Geometry: see drawing. Coordinates: mm, zero at the bounding-box minimum. Coordinates: 2 decimals unless noted, no trailing zeros. Write each loop counter-clockwise with the first axis right and the second up, starting at its lowest first coordinate (ties: lowest second). Pieces come first, ordered by that corner, then holes. Notation, with made-up numbers: (37, 53.25) - (53, 53.25) arc R25 cw to (53, 66.25) - close; hole circle Ø4 at (11.25, 1.25). An arc over 180 degrees is marked (long way). One line per question, with ' | ' between items. Start each with the question number.
1) Section query B-B on y = 1.8. Return loops of the section in (x, z).
2) Line query: line 1 (Z direction, x = 9, y = 3.4); line 2 (X direction, y = 4.7, z = 3); line 3 (Z direction, x = 44.5, y = 3.35). Output: solid intervals per line, ascending.
3) Section query D-D on x = 36.5. Return loops of the section in (y, z), and give its area (3 significant figures).
4) Section query A-A on x = 10. Return loops of the section in (y, z), and give its area (3 significant figures).
5) First-contact query: P1, Ø1.5, axis at y = 2.5, z = 34.5, coming from the -X side; P2, Ø2.5, axis at y = 2.5, z = 22, coming from the +X side. Flat tips, straight axial feed; report the tip coordinate or a pass-through.
6) Section query C-C on z = 28.5. Return loops of the section in (x, y), and give its area (3 significant figures).
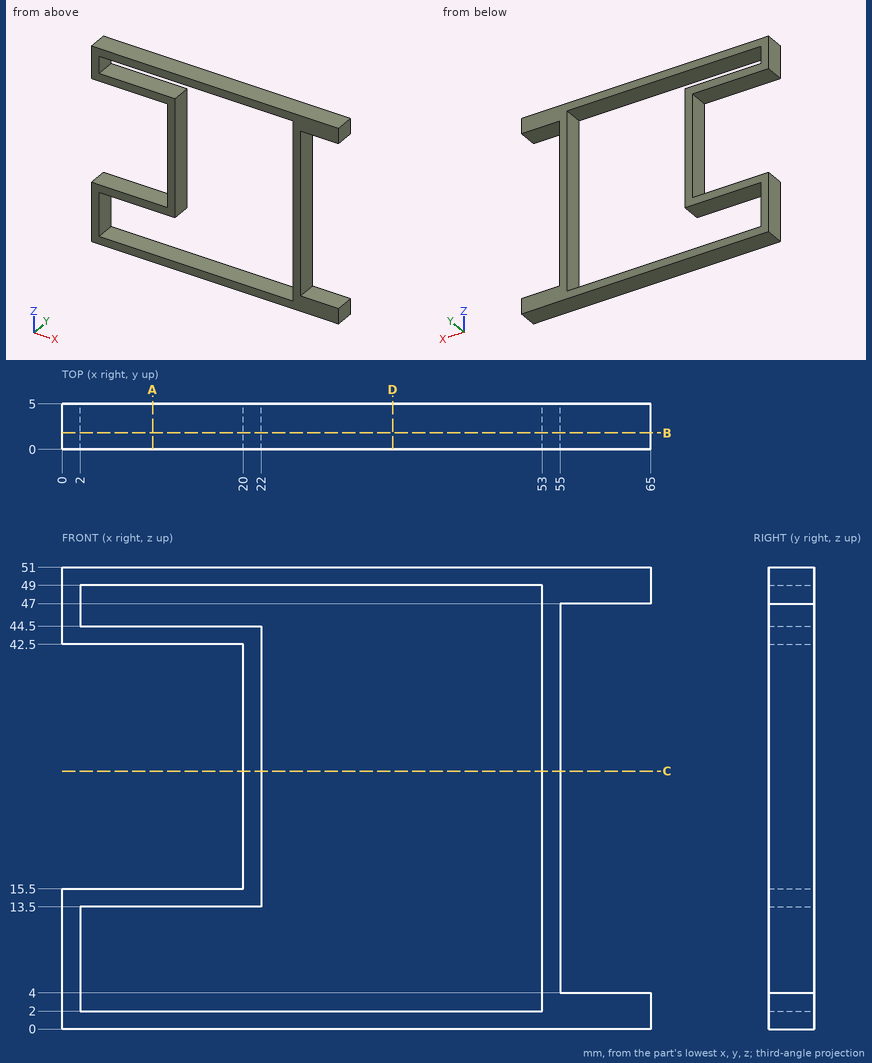
Answer key:
1) outline: (0, 0) - (65, 0) - (65, 4) - (55, 4) - (55, 47) - (65, 47) - (65, 51) - (0, 51) - (0, 42.5) - (20, 42.5) - (20, 15.5) - (0, 15.5) - close; hole (2, 2) - (53, 2) - (53, 49) - (2, 49) - (2, 44.5) - (22, 44.5) - (22, 13.5) - (2, 13.5) - close
2) line 1: 0 to 2, 13.5 to 15.5, 42.5 to 44.5, 49 to 51 | line 2: 0 to 2, 53 to 65 | line 3: 0 to 2, 49 to 51
3) outline: (0, 0) - (5, 0) - (5, 2) - (0, 2) - close; (0, 49) - (5, 49) - (5, 51) - (0, 51) - close | area: 20.0 mm²
4) outline: (0, 0) - (5, 0) - (5, 2) - (0, 2) - close; (0, 13.5) - (5, 13.5) - (5, 15.5) - (0, 15.5) - close; (0, 42.5) - (5, 42.5) - (5, 44.5) - (0, 44.5) - close; (0, 49) - (5, 49) - (5, 51) - (0, 51) - close | area: 40.0 mm²
5) P1: x = 20 | P2: x = 55
6) outline: (20, 0) - (22, 0) - (22, 5) - (20, 5) - close; (53, 0) - (55, 0) - (55, 5) - (53, 5) - close | area: 20.0 mm²
